Can you work these out from the model? Positions are in its coordinate system, mm. A direction names the side the tool comes from. Coordinates: 2 decimals unless noted, no trailing zeros. Order: outer loops, then holes, each group sorted by start corner. A loop starts at its lowest first (then second) coordinate and runs counter-clockwise, first axis right, second up.
```python
from build123d import *


with BuildPart() as f1:
    # F0 (on Front) → F1 (revolve)
    with BuildSketch(Plane.XZ):
        with BuildLine():
            Line((18.64121, 0), (0, 0))
            Line((0, 0), (0, -25.406862))
            Line((0, -25.406862), (25.393533, -25.406862))
            Line((25.393533, -25.406862), (25.393533, -44.454585))
            ThreePointArc((25.393533, -44.454585), (26.323469, -46.699649), (28.568533, -47.629585))
            Line((28.568533, -47.629585), (29.843302, -47.629585))
            Line((29.843302, -47.629585), (31.11807, -46.364747))
            Line((31.11807, -46.364747), (31.11807, -18.42168))
            Line((31.11807, -18.42168), (28.557492, -18.42168))
            Line((28.557492, -18.42168), (28.557492, -13.31171))
            Line((28.557492, -13.31171), (18.64121, -13.31171))
            Line((18.64121, -13.31171), (18.64121, 0))
        make_face()
    revolve(axis=Axis((9.320605, 0, 0), (-1, 0, 0)))


solid = f1.part
```
1. Please list where these lines run through material, in increasing order: probe 1 along Z at (x, y) = (29, 0); probe 2 along Y at (x, z) = (30.5, 0); probe 3 along X at (y, z) = (15, 5).
Completed:
probe 1: z = -47.63 to -18.42, 18.42 to 47.63
probe 2: y = -46.98 to -18.42, 18.42 to 46.98
probe 3: x = 0 to 28.56
2. On a 3-axis mill with a long thin cutter (end or side, diameter ignored), from which of +Z, -Z, +X, -X, +Y, -Y can I reach the whole of each face in a straight line? I mean faces 5 (the flat face through (0, 0, 0)), 6 (the flat face through (18.641, 0, 0)), 7 (the flat face through (25.394, 19, 19)). Say none if no direction works.
Completed:
face 5: +Z, -Z, -X, +Y, -Y
face 6: +X
face 7: -X
3. Thinking about a two-plate mould opening in Z: for faces 1 (the flat face through (28.557, -9.6, -9.5)), 2 (the flat face through (31.118, -1, -20)), 3 (the cylindrical face through (29.21, -14.31, -45.43)), 4 (the cylindrical face through (29.82, -5.53, -17.57)), which applies, pulls with the +Z half, pulls with the -Z half, needs draft (parallel to the pull), parting line crosses it, or undercut?
Completed:
face 1: undercut
face 2: needs draft
face 3: parting line crosses it
face 4: undercut
4. Imagine slicing it at C-C on x = 21. Please give me the cut outline in (y, z), then the cut area to 3 significant figures.
Completed:
outline: circle Ø50.81 at (0, 0); hole circle Ø26.62 at (0, 0)
area: 1,470 mm2
5. Imagine slicing it at D-D on x = 13.5. Please give me the cut outline in (y, z), then the cut area to 3 significant figures.
Completed:
outline: circle Ø50.81 at (0, 0)
area: 2,030 mm2
6. I'm going to push flat-ended pins straight in: pin 1 (10 mm diameter, centred on y = -35.5, z = -6.5, fed in from -X); pin 2 (4 mm diameter, centred on x = 10, y = 3.5, fed in from -Z); pin 3 (6 mm diameter, centred on x = 21.5, z = -22.5, fed in from +Y). Where does each tip first touch, or does it pass through?
Completed:
pin 1: stops at x = 25.39
pin 2: stops at z = -25.36
pin 3: stops at y = 16.29
